Answer from the drawing. Dimensions are ordinates in mm from the lowest x, y and z of the part. A direction names the side the tool comes from. Give positions to 0.01 mm unless a question says otherwise; leave off trailing zeros. Write each loop counter-clockwise with the first axis right and the second up, starting at its lowest first coordinate (ties: lowest second). Pieces come first, ordered by that corner, then holes. Notation, with made-up numbers: (16.5, 44) -> (59.5, 44) arc R20 cw to (59.5, 60) -> close; hole circle Ø3 at (80.5, 10.5). An arc over 180 degrees is marked (long way). Write item = value, one per line.
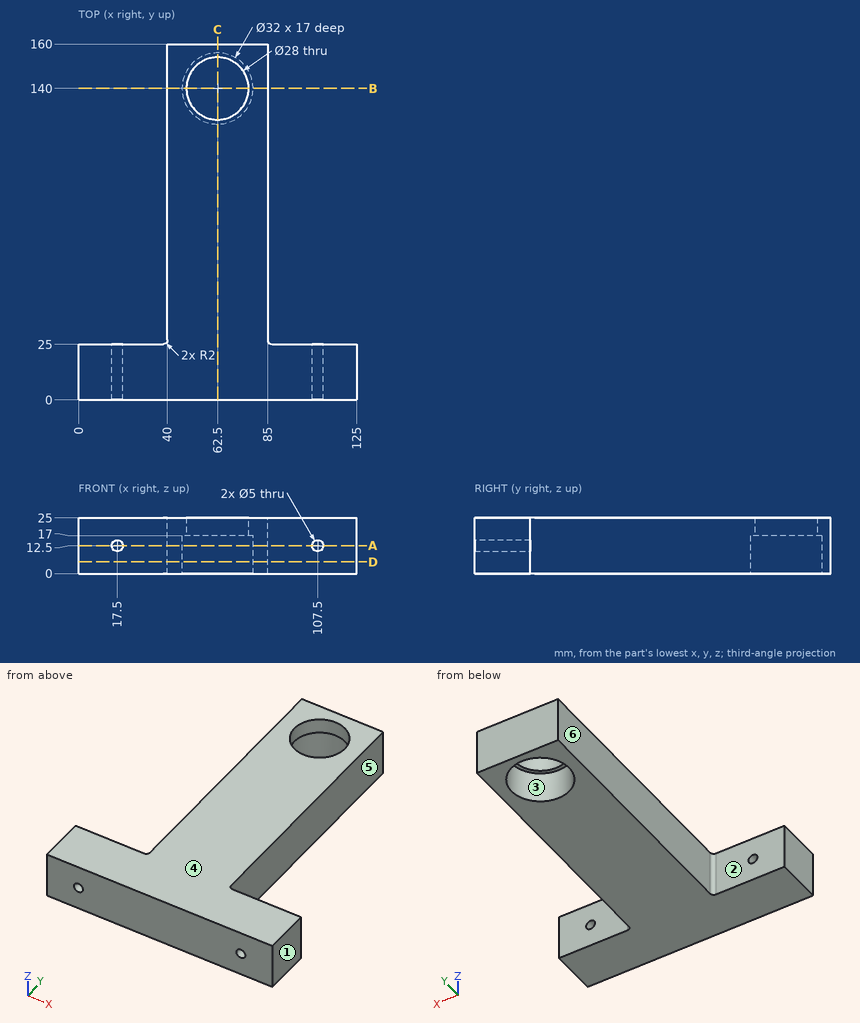
(1) Consider L1, parallel to X at y = 9, z = 12.5; L2, parallel to Y at x = 62.5, z = 20.75; L3, parallel to X at y = 83, z = 12. Determine where each line is inside the solid, lowest interval first.
Checks:
L1 = 0 to 15, 20 to 105, 110 to 125
L2 = 0 to 126, 154 to 160
L3 = 40 to 85
(2) The part is cut by section B-B on y = 140. Determine the outline of the cut face in (x, z).
Checks:
outline = (40, 0) -> (46.5, 0) -> (46.5, 17) -> (48.5, 17) -> (48.5, 25) -> (40, 25) -> close; (76.5, 17) -> (78.5, 17) -> (78.5, 0) -> (85, 0) -> (85, 25) -> (76.5, 25) -> close
(3) The part is cut by section D-D on z = 5.25. Determine the outline of the cut face in (x, y).
Checks:
outline = (0, 0) -> (125, 0) -> (125, 25) -> (87, 25) arc R2 cw to (85, 27) -> (85, 160) -> (40, 160) -> (40, 27) arc R2 cw to (38, 25) -> (0, 25) -> close; hole circle Ø32 at (62.5, 140)
(4) The part is cut by section C-C on x = 62.5. Determine the outline of the cut face in (y, z).
Checks:
outline = (0, 0) -> (124, 0) -> (124, 17) -> (126, 17) -> (126, 25) -> (0, 25) -> close; (154, 17) -> (156, 17) -> (156, 0) -> (160, 0) -> (160, 25) -> (154, 25) -> close
(5) A tool of negligible diameter and unlimited length cuts with its end or side. For the marked faces 4, 5 and 6, from which of +Z, -Z, +X, -X, +Y, -Y can it reach the whole face along a straight path? Write none if from no direction.
Checks:
face_4 = +Z, +X, -X, +Y, -Y
face_5 = +Z, -Z, +X, +Y
face_6 = +Z, -Z, -X, +Y
(6) Given P1, Ø12, axis at y = 97.5, z = 18, coming from the +X side; P2, Ø7.5, axis at y = 72.5, z = 12.5, coming from the -X side; P3, Ø8, axis at x = 25.5, z = 10, coming from the -Y side; P4, Ø12.5, axis at x = 15, z = 12, coming from the +Y side, each flat-ended and moving along its own axis, determine where each tip first touches the part or whether it passes through.
Checks:
P1 = 85
P2 = 40
P3 = 0
P4 = 25
(7) For a pull along X with two mould halves and no side action, classify the marked faces 1, 2 and 3 as released by +X, released by -X, zero draft, split by the parting line, or undercut.
Checks:
face_1 = released by +X
face_2 = zero draft
face_3 = undercut
(8) The part is cut by section A-A on z = 12.5. Determine the outline of the cut face in (x, y).
Checks:
outline = (0, 0) -> (15, 0) -> (15, 25) -> (0, 25) -> close; (20, 0) -> (105, 0) -> (105, 25) -> (87, 25) arc R2 cw to (85, 27) -> (85, 160) -> (40, 160) -> (40, 27) arc R2 cw to (38, 25) -> (20, 25) -> close; (110, 0) -> (125, 0) -> (125, 25) -> (110, 25) -> close; hole circle Ø32 at (62.5, 140)
